Could you check a few things on this model? Use its own coordinates, in mm. Face numbers are marked on the shaded views. A direction names the side the tool comes from. Coordinates: 2 decimals unless noted, no trailing zeros. Write each loop counter-clockwise with the first axis right and the second up, starting at its lowest first coordinate (ties: lowest second). Pieces come first, ordered by that corner, then holes. Notation, with made-up numbers: (63, 62) - (98, 62) arc R8 ccw to (98, 67) - close; hole circle Ø7 at (22, 25.5). An arc over 180 degrees is marked (long way). Answer as a JSON object with one key per item and string values. Group by question number.
1) We'd pull the mould along Z, two halves only. Please class the marked faces 3, 4, 5 and 6: released by +Z, released by -Z, zero draft, split by the parting line, or undercut.
2) If we section it at D-D (x = -131.5): Write out the boundary of the cut face in (y, z).
3) If we section it at C-C (z = -368.75): Write out the boundary of the cut face in (x, y).
4) On a 3-axis mill with a long thin cutter (end or side, diameter ignored), from which of +Z, -Z, +X, -X, +Y, -Y can I reach the whole of each face in a straight line? I mean the marked faces 1 and 2. Say none if no direction works.
5) If we section it at A-A (x = -116.5): Write out the boundary of the cut face in (y, z), plus the area to 3 significant figures.
6) If we section it at B-B (y = 22): Write out the boundary of the cut face in (x, z), plus the area to 3 significant figures.
7) Will these pins go through, and if not, where does the flat tip stop? pin 1 Ø3 at (x, y) = (-123, 30.5) entering from -Z; pin 2 Ø8 at (x, y) = (-120, 34) entering from +Z.
8) Please list where these lines run through material, in increasing order: line 1 along Y through (x, z) = (-117, -367.5); line 2 along X through (y, z) = (32, -372); line 3 along X through (y, z) = (30.5, -367.25) (3 decimals).
```python
from build123d import *

# Parameters (mm, degrees)
BOSS_EXTRUDE1_DEPTH   = 45
SKETCH1_R             = 7.6
BOSS_EXTRUDE1_2_DEPTH = 45
BOSS_EXTRUDE1_3_DEPTH = 45
SKETCH1_3_R           = 7.6
BOSS_EXTRUDE2_DEPTH   = 6.4
SKETCH2_W             = 43.8
SKETCH2_H             = 15.2
BOSS_EXTRUDE3_DEPTH   = 6.4


with BuildPart() as part:
    # Sketch1 → Boss-Extrude1 (new body)
    with BuildSketch(Plane(origin=(0, 0, 0), x_dir=(1, 0, 0), z_dir=(0, 1, 0))):
        with BuildLine():
            Line((-107.578947368, 374.605263158), (-115.115713053, 374.605263158))
            ThreePointArc((-115.115713053, 374.605263158), (-113.707690956, 370.920613869), (-113.228947368, 367.005263158))
            ThreePointArc((-113.228947368, 367.005263158), (-113.707690956, 363.089912447), (-115.115713053, 359.405263158))
            Line((-115.115713053, 359.405263158), (-107.578947368, 359.405263158))
            Line((-107.578947368, 359.405263158), (-107.578947368, 374.605263158))
        make_face()
    extrude(amount=BOSS_EXTRUDE1_DEPTH)



with BuildPart() as body_2:
    # Sketch1 → Boss-Extrude1 2 (new body)
    with BuildSketch(Plane(origin=(0, 0, 0), x_dir=(1, 0, 0), z_dir=(0, 1, 0))):
        with Locations((-129.478947368, 367.005263158)):
            Circle(SKETCH1_R)
    extrude(amount=BOSS_EXTRUDE1_2_DEPTH)


with BuildPart() as body_3:
    # Sketch1 → Boss-Extrude1 3 (new body)
    with BuildSketch(Plane(origin=(0, 0, 0), x_dir=(1, 0, 0), z_dir=(0, 1, 0))):
        with BuildLine():
            Line((-143.842181684, 374.605263158), (-151.378947368, 374.605263158))
            Line((-151.378947368, 374.605263158), (-151.378947368, 359.405263158))
            Line((-151.378947368, 359.405263158), (-143.842181684, 359.405263158))
            ThreePointArc((-143.842181684, 359.405263158), (-145.728947368, 367.005263158), (-143.842181684, 374.605263158))
        make_face()
    extrude(amount=BOSS_EXTRUDE1_3_DEPTH)


with BuildPart() as part_1:
    add(part.part)

    add(body_2.part)  # Boss-Extrude2 merges body 2

    add(body_3.part)  # Boss-Extrude2 merges body 3
    # Sketch1_3 → Boss-Extrude2 (add)
    with BuildSketch(Plane(origin=(0, 0, 0), x_dir=(1, 0, 0), z_dir=(0, 1, 0))):
        with BuildLine():
            Line((-143.842181684, 374.605263158), (-151.378947368, 374.605263158))
            Line((-151.378947368, 374.605263158), (-151.378947368, 359.405263158))
            Line((-151.378947368, 359.405263158), (-143.842181684, 359.405263158))
            ThreePointArc((-143.842181684, 359.405263158), (-145.728947368, 367.005263158), (-143.842181684, 374.605263158))
        make_face()
        with BuildLine():
            Line((-129.478947368, 374.605263158), (-143.842181684, 374.605263158))
            ThreePointArc((-143.842181684, 374.605263158), (-145.728947368, 367.005263158), (-143.842181684, 359.405263158))
            Line((-143.842181684, 359.405263158), (-129.478947368, 359.405263158))
            ThreePointArc((-129.478947368, 359.405263158), (-137.078947368, 367.005263158), (-129.478947368, 374.605263158))
        make_face()
        with BuildLine():
            Line((-115.115713053, 374.605263158), (-129.478947368, 374.605263158))
            ThreePointArc((-129.478947368, 374.605263158), (-124.104935831, 372.379274695), (-121.878947368, 367.005263158))
            ThreePointArc((-121.878947368, 367.005263158), (-124.104935831, 361.631251621), (-129.478947368, 359.405263158))
            Line((-129.478947368, 359.405263158), (-115.115713053, 359.405263158))
            ThreePointArc((-115.115713053, 359.405263158), (-113.707690956, 363.089912447), (-113.228947368, 367.005263158))
            ThreePointArc((-113.228947368, 367.005263158), (-113.707690956, 370.920613869), (-115.115713053, 374.605263158))
        make_face()
        with Locations((-129.478947368, 367.005263158)):
            Circle(SKETCH1_3_R)
        with BuildLine():
            Line((-107.578947368, 374.605263158), (-115.115713053, 374.605263158))
            ThreePointArc((-115.115713053, 374.605263158), (-113.707690956, 370.920613869), (-113.228947368, 367.005263158))
            ThreePointArc((-113.228947368, 367.005263158), (-113.707690956, 363.089912447), (-115.115713053, 359.405263158))
            Line((-115.115713053, 359.405263158), (-107.578947368, 359.405263158))
            Line((-107.578947368, 359.405263158), (-107.578947368, 374.605263158))
        make_face()
    extrude(amount=BOSS_EXTRUDE2_DEPTH)

    # Sketch2 → Boss-Extrude3 (add)
    with BuildSketch(Plane(origin=(0, 45, 0), x_dir=(1, 0, 0), z_dir=(0, 1, 0))):
        with Locations((-129.478947368, 367.005263158)):
            Rectangle(SKETCH2_W, SKETCH2_H)
    extrude(amount=-BOSS_EXTRUDE3_DEPTH)


solid = part_1.part
```
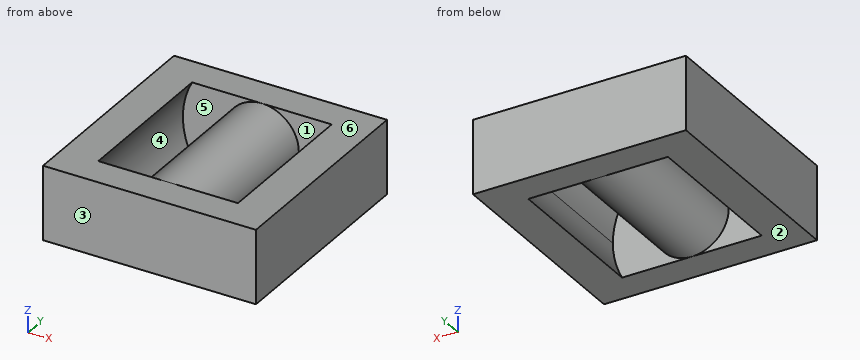
Here are the results:
{
 "1": {"face 3": "zero draft", "face 4": "undercut", "face 5": "undercut", "face 6": "released by +Z"},
 "2": {"outline": "(0, -374.61) - (6.4, -374.61) - (6.4, -374.33) - (38.6, -374.33) - (38.6, -374.61) - (45, -374.61) - (45, -359.41) - (38.6, -359.41) - (38.6, -359.68) - (6.4, -359.68) - (6.4, -359.41) - (0, -359.41) - close"},
 "3": {"outline": "(-151.38, 0) - (-107.58, 0) - (-107.58, 45) - (-151.38, 45) - close; hole (-145.64, 6.4) - (-136.88, 6.4) - (-136.88, 38.6) - (-145.64, 38.6) - close; hole (-122.08, 6.4) - (-113.32, 6.4) - (-113.32, 38.6) - (-122.08, 38.6) - close"},
 "4": {"face 1": "none", "face 2": "-Z, +X, -X, +Y, -Y"},
 "5": {"outline": "(0, -374.61) - (6.4, -374.61) - (6.4, -359.41) - (0, -359.41) - close; (38.6, -374.61) - (45, -374.61) - (45, -359.41) - (38.6, -359.41) - close", "area": "195 mm²"},
 "6": {"outline": "(-151.38, -374.61) - (-143.84, -374.61) arc R16.25 cw to (-143.84, -359.41) - (-151.38, -359.41) - close; circle Ø15.2 at (-129.48, -367.01); (-115.12, -374.61) - (-107.58, -374.61) - (-107.58, -359.41) - (-115.12, -359.41) arc R16.25 cw to start", "area": "372 mm²"},
 "7": {"pin 1": "stops at z = -372.75", "pin 2": "stops at z = -361.74"},
 "8": {"line 1": "y = 0 to 6.4, 38.6 to 45", "line 2": "x = -151.38 to -144.94, -135.21 to -123.75, -114.02 to -107.58", "line 3": "x = -151.379 to -145.727, -137.075 to -121.883, -113.231 to -107.579"}
}
